```python
from build123d import *

# Parameters (mm, degrees)
SKETCH_W           = 280
SKETCH_H           = 110
SKETCH_R           = 37.75
SKETCH_R_2         = 26.25
SKETCH_R_3         = 1.75
PAD_DEPTH          = 8
SKETCH001_R        = 2.1
POCKET_DEPTH       = 8
POLARPATTERN_COUNT = 6
SKETCH002_R        = 47
SKETCH002_R_2      = 37.75
POCKET001_DEPTH    = 4.5
SKETCH003_R        = 26.25
POCKET002_DEPTH    = 4.3
SKETCH004_R        = 1.75
POCKET003_DEPTH    = 8
FILLET002_R        = 4


with BuildPart() as part:
    # Sketch → Pad (new body)
    with BuildSketch(Plane.XY):
        Rectangle(SKETCH_W, SKETCH_H)
        Circle(SKETCH_R, mode=Mode.SUBTRACT)
        with Locations((93.5, 0)):
            Circle(SKETCH_R_2, mode=Mode.SUBTRACT)
        with Locations((-93.5, 0)):
            Circle(SKETCH_R_2, mode=Mode.SUBTRACT)
        with Locations((116.516326, -23.016326)):
            Circle(SKETCH_R_3, mode=Mode.SUBTRACT)
        with Locations((116.516326, 23.016326)):
            Circle(SKETCH_R_3, mode=Mode.SUBTRACT)
        with Locations((70.483674, 23.016326)):
            Circle(SKETCH_R_3, mode=Mode.SUBTRACT)
        with Locations((70.483674, -23.016326)):
            Circle(SKETCH_R_3, mode=Mode.SUBTRACT)
        with Locations((-116.516326, 23.016326)):
            Circle(SKETCH_R_3, mode=Mode.SUBTRACT)
        with Locations((-70.483674, 23.016326)):
            Circle(SKETCH_R_3, mode=Mode.SUBTRACT)
        with Locations((-70.483674, -23.016326)):
            Circle(SKETCH_R_3, mode=Mode.SUBTRACT)
        with Locations((-116.516326, -23.016326)):
            Circle(SKETCH_R_3, mode=Mode.SUBTRACT)
    extrude(amount=PAD_DEPTH)

    # Sketch001 (on Face17 of Pad) → Pocket (cut)
    with BuildSketch(Plane.XY.offset(8)):
        with Locations((42, 0)):
            Circle(SKETCH001_R)
    pocket = extrude(amount=-POCKET_DEPTH, mode=Mode.SUBTRACT)

    # PolarPattern: Pocket ×6 about axis
    polarpattern_axis = Axis((0, 0, 8), (0, 0, 1))
    for i in range(1, POLARPATTERN_COUNT):
        add(pocket.rotate(polarpattern_axis, i * 360 / POLARPATTERN_COUNT), mode=Mode.SUBTRACT)

    # Sketch002 (on Face5 of PolarPattern) → Pocket001 (cut)
    with BuildSketch(Plane.XY.offset(8)):
        Circle(SKETCH002_R)
        Circle(SKETCH002_R_2, mode=Mode.SUBTRACT)
    extrude(amount=-POCKET001_DEPTH, mode=Mode.SUBTRACT)

    # Sketch003 (on Face5 of Pocket001) → Pocket002 (cut)
    with BuildSketch(Plane.XY.offset(8)):
        with BuildLine():
            Line((-119.25, 28.75), (-67.75, 28.75))
            ThreePointArc((-64.75, 25.75), (-65.62868, 27.87132), (-67.75, 28.75))
            Line((-64.75, 25.75), (-64.75, -25.75))
            ThreePointArc((-67.75, -28.75), (-65.62868, -27.87132), (-64.75, -25.75))
            Line((-67.75, -28.75), (-119.25, -28.75))
            ThreePointArc((-122.25, -25.75), (-121.37132, -27.87132), (-119.25, -28.75))
            Line((-122.25, -25.75), (-122.25, 25.75))
            ThreePointArc((-119.25, 28.75), (-121.37132, 27.87132), (-122.25, 25.75))
        make_face()
        with Locations((-93.5, 0)):
            Circle(SKETCH003_R, mode=Mode.SUBTRACT)
        with BuildLine():
            Line((67.75, 28.75), (119.25, 28.75))
            ThreePointArc((122.25, 25.75), (121.37132, 27.87132), (119.25, 28.75))
            Line((122.25, 25.75), (122.25, -25.75))
            ThreePointArc((119.25, -28.75), (121.37132, -27.87132), (122.25, -25.75))
            Line((119.25, -28.75), (67.75, -28.75))
            ThreePointArc((64.75, -25.75), (65.62868, -27.87132), (67.75, -28.75))
            Line((64.75, -25.75), (64.75, 25.75))
            ThreePointArc((67.75, 28.75), (65.62868, 27.87132), (64.75, 25.75))
        make_face()
        with Locations((93.5, 0)):
            Circle(SKETCH003_R, mode=Mode.SUBTRACT)
    extrude(amount=-POCKET002_DEPTH, mode=Mode.SUBTRACT)

    # Sketch004 (on Face5 of Pocket002) → Pocket003 (cut)
    with BuildSketch(Plane.XY.offset(8)):
        with Locations((-135, 50)):
            Circle(SKETCH004_R)
        with Locations((-135, -50)):
            Circle(SKETCH004_R)
        with Locations((135, -50)):
            Circle(SKETCH004_R)
        with Locations((135, 50)):
            Circle(SKETCH004_R)
    extrude(amount=-POCKET003_DEPTH, mode=Mode.SUBTRACT)

    # Fillet002
    fillet002_edges = [part.edges().sort_by_distance(p)[0] for p in [
        (140, -55, 4),
        (-140, -55, 4),
        (-140, 55, 4),
        (140, 55, 4),
    ]]
    fillet(fillet002_edges, radius=FILLET002_R)


solid = part.part
```
Here's how the part is built. I have some questions about the finished solid (model axes, mm). A direction names the side the tool comes from. Give positions to 0.01 mm unless a question says otherwise; leave off trailing zeros. Write each loop counter-clockwise with the first axis right and the second up, starting at its lowest first coordinate (ties: lowest second). Pieces come first, ordered by that corner, then holes.
(1) Will these pins go through, and if not, where does the flat tip stop? pin 1 (5.5 mm diameter, centred on x = -135, y = -50, fed in from +Z); pin 2 (4 mm diameter, centred on x = -116.52, y = 23.02, fed in from +Z).
Output values:
pin 1: stops at z = 8
pin 2: stops at z = 3.7
(2) Imagine slicing it at C-C, the plane y = -6. Write out the boundary of the cut face in (x, z).
Output values:
outline: (-140, 0) - (-119.06, 0) - (-119.06, 3.7) - (-122.25, 3.7) - (-122.25, 8) - (-140, 8) - close; (-67.94, 0) - (-37.27, 0) - (-37.27, 3.5) - (-46.62, 3.5) - (-46.62, 8) - (-64.75, 8) - (-64.75, 3.7) - (-67.94, 3.7) - close; (37.27, 0) - (67.94, 0) - (67.94, 3.7) - (64.75, 3.7) - (64.75, 8) - (46.62, 8) - (46.62, 3.5) - (37.27, 3.5) - close; (119.06, 0) - (140, 0) - (140, 8) - (122.25, 8) - (122.25, 3.7) - (119.06, 3.7) - close
(3) Imagine slicing it at B-B, the plane z = 5. Count the separate pieces of the cut face and the enclosed holes in it, and give its area (3 significant figures).
Output values:
separate pieces: 1
enclosed holes: 7
area: 17,200 mm2
(4) Thinking about a two-plate mould opening in X: for faces 3 (the face through (140, -1, 4)), 4 (the face through (-140, -1, 4)), 5 (the face through (-33, 25, 0)), 6 (the face through (-100, 26, 3.7)), which applies, pulls with the +X half, pulls with the -X half, needs draft (parallel to the pull), parting line crosses it, or undercut?
Output values:
face 3: pulls with the +X half
face 4: pulls with the -X half
face 5: needs draft
face 6: undercut
(5) On a 3-axis mill with a long thin cutter (end or side, diameter ignored), from which of +Z, -Z, +X, -X, +Y, -Y can I reach the whole of each face in a straight line? I mean faces 1 (the face through (67.275, 1.154, 1.824)), 2 (the face through (0, 39, 3.5)). Say none if no direction works.
Output values:
face 1: +Z, -Z
face 2: +Z
(6) If I drill on L1, parallel to Y at x = -92, z = 2.25; L2, parallel to Y at x = -87, z = 7.75; L3, parallel to X at y = -16.5, z = 1.75, over which ranges is the centre line in solid material (lowest first)?
Output values:
L1: y = -55 to -26.21, 26.21 to 55
L2: y = -55 to -28.75, 28.75 to 55
L3: x = -140 to -113.92, -73.08 to -33.95, 33.95 to 73.08, 113.92 to 140
(7) Imagine slicing it at D-D, the plane y = -31.5. Write out the boundary of the cut face in (x, z).
Output values:
outline: (-140, 0) - (-20.8, 0) - (-20.8, 3.5) - (-34.88, 3.5) - (-34.88, 8) - (-140, 8) - close; (20.8, 0) - (140, 0) - (140, 8) - (34.88, 8) - (34.88, 3.5) - (20.8, 3.5) - close
(8) Imagine slicing it at A-A, the plane x = 0. Write out the boundary of the cut face in (y, z).
Output values:
outline: (-55, 0) - (-37.75, 0) - (-37.75, 3.5) - (-47, 3.5) - (-47, 8) - (-55, 8) - close; (37.75, 0) - (55, 0) - (55, 8) - (47, 8) - (47, 3.5) - (37.75, 3.5) - close
